Geometry check sheet. Reference: the model listing, model coordinates, mm. A direction names the side the tool comes from. Round coordinates to 2 decimals unless told otherwise and drop trailing zeros. Order: outer loops, then holes, each group sorted by start corner. A loop starts at its lowest first (then second) coordinate and runs counter-clockwise, first axis right, second up. Notation, with made-up numbers: (66, 52) -> (104, 52) arc R24 cw to (104, 79) -> close; hole circle Ø8 at (50, 77). An arc over 180 degrees is marked (long way). Answer as a JSON object with one key per item and string values. Group by question number.
from build123d import *

# Parameters (mm, degrees)
SKETCH_1_W          = 32
SKETCH_1_H          = 28
EXTRUDE_1_DEPTH     = 1.2
SKETCH_2_W          = 32
SKETCH_2_H          = 17.6
EXTRUDE_2_DEPTH     = 1.8
SKETCH_3_R          = 1.1
CUT_EXTRUDE_1_DEPTH = 43.558665393
SKETCH_4_R          = 0.4
EXTRUDE_3_DEPTH     = 10
SKETCH_5_W          = 20.3
SKETCH_5_H          = 2.5
EXTRUDE_4_DEPTH     = 2.5


with BuildPart() as part:
    # 草图1 → 凸台-拉伸1 (new body)
    with BuildSketch(Plane(origin=(0, 0, 0), x_dir=(1, 0, 0), z_dir=(0, 1, 0))):
        with Locations((16, 14)):
            Rectangle(SKETCH_1_W, SKETCH_1_H)
    extrude(amount=EXTRUDE_1_DEPTH)

    # 草图2 → 凸台-拉伸2 (add)
    with BuildSketch(Plane(origin=(0, 1.2, 0), x_dir=(1, 0, 0), z_dir=(0, 1, 0))):
        with Locations((16, 14)):
            Rectangle(SKETCH_2_W, SKETCH_2_H)
    extrude(amount=EXTRUDE_2_DEPTH)

    # 草图3 → 切除-拉伸1 (cut, through all)
    with BuildSketch(Plane(origin=(0, 1.2, 0), x_dir=(1, 0, 0), z_dir=(0, 1, 0))):
        with Locations(Location((2.75, 25.5, 0), (0, 0, 270))):
            Circle(SKETCH_3_R)
        with Locations(Location((2.75, 2.5, 0), (0, 0, 90))):
            Circle(SKETCH_3_R)
        with Locations(Location((29.25, 2.5, 0), (0, 0, 270))):
            Circle(SKETCH_3_R)
        with Locations(Location((29.25, 25.5, 0), (0, 0, 90))):
            Circle(SKETCH_3_R)
    extrude(amount=-CUT_EXTRUDE_1_DEPTH, mode=Mode.SUBTRACT)

    # 草图4 → 凸台-拉伸3 (add)
    with BuildSketch(Plane.XZ):
        with Locations(Location((7.11, -1.27, 0), (0, 0, 270))):
            Circle(SKETCH_4_R)
        with Locations(Location((9.65, -1.27, 0), (0, 0, 270))):
            Circle(SKETCH_4_R)
        with Locations(Location((12.19, -1.27, 0), (0, 0, 270))):
            Circle(SKETCH_4_R)
        with Locations(Location((14.73, -1.27, 0), (0, 0, 270))):
            Circle(SKETCH_4_R)
        with Locations(Location((17.27, -1.27, 0), (0, 0, 270))):
            Circle(SKETCH_4_R)
        with Locations(Location((19.81, -1.27, 0), (0, 0, 270))):
            Circle(SKETCH_4_R)
        with Locations(Location((22.35, -1.27, 0), (0, 0, 270))):
            Circle(SKETCH_4_R)
        with Locations(Location((24.89, -1.27, 0), (0, 0, 270))):
            Circle(SKETCH_4_R)
    extrude(amount=EXTRUDE_3_DEPTH)

    # 草图5 → 凸台-拉伸4 (add)
    with BuildSketch(Plane.XZ):
        with Locations((16, -1.25)):
            Rectangle(SKETCH_5_W, SKETCH_5_H)
    extrude(amount=EXTRUDE_4_DEPTH)


solid = part.part
Item 1: Mould release check, pull along X, two halves, no side actions. Record for faces 1 (the flat face through (26.15, -1, -1)), 2 (the cylindrical face through (10.047, -6.198, -1.218)), 3 (the flat face through (5.85, -1, -1)), 4 (the flat face through (16, 0, 0)): pulls with the +X half, pulls with the -X half, needs draft (parallel to the pull), parting line crosses it, or undercut.
Item 2: Sectioned sample at D-D, the plane x = 12.19. Enter the section's corners in (y, z).
Item 3: Set-up check for faces 5 (the flat face through (16, 2, -22.8)), 6 (the cylindrical face through (2.8, 0.6, -26.6)), 7 (the flat face through (16, -1, -2.5)), 8 (the cylindrical face through (15.127, -6.198, -1.218)), 9 (the flat face through (16, 1.2, -3)): record each of +Z, -Z, +X, -X, +Y, -Y from which the full face is reachable in a straight line by a thin tool's end or side.
Item 4: Sectioned sample at B-B, the plane y = -6.25. Enter the section's corners in (x, z).
Item 5: Depth check by flat-ended pin: pin 1 Ø1.2 at (y, z) = (-1, -2) entering from +X; pin 2 Ø3.5 at (x, z) = (29.25, -2.5) entering from +Y; pin 3 Ø10 at (x, z) = (8, -8) entering from -Y. Enter the tip coordinate at first touch or a pass-through.
Item 6: Thickness scan on L1, parallel to X at y = 0.75, z = -25.5; L2, parallel to Y at x = 13, z = -11.5; L3, parallel to Z at x = 10.5, y = 1.5. Record the ranges inside material, lowest first.
Item 7: Sectioned sample at A-A, the plane x = 29.25. Enter the section's corners in (y, z).
Item 8: Sectioned sample at C-C, the plane z = -25.5. Enter the section's corners in (x, y).
Result:
{
 "1": {"face 1": "pulls with the +X half", "face 2": "undercut", "face 3": "pulls with the -X half", "face 4": "needs draft"},
 "2": {"outline": "(-10, -1.67) -> (-2.5, -1.67) -> (-2.5, -2.5) -> (0, -2.5) -> (0, -28) -> (1.2, -28) -> (1.2, -22.8) -> (3, -22.8) -> (3, -5.2) -> (1.2, -5.2) -> (1.2, 0) -> (-2.5, 0) -> (-2.5, -0.87) -> (-10, -0.87) -> close"},
 "3": {"face 5": "-Z, +X, -X, +Y", "face 6": "+Y, -Y", "face 7": "-Z, +X, -X, -Y", "face 8": "-Y", "face 9": "+Z, +X, -X, +Y"},
 "4": {"outline": "circle Ø0.8 at (7.11, -1.27); circle Ø0.8 at (9.65, -1.27); circle Ø0.8 at (12.19, -1.27); circle Ø0.8 at (14.73, -1.27); circle Ø0.8 at (17.27, -1.27); circle Ø0.8 at (19.81, -1.27); circle Ø0.8 at (22.35, -1.27); circle Ø0.8 at (24.89, -1.27)"},
 "5": {"pin 1": "stops at x = 26.15", "pin 2": "stops at y = 1.2", "pin 3": "stops at y = 0"},
 "6": {"L1": "x = 0 to 1.65, 3.85 to 28.15, 30.35 to 32", "L2": "y = 0 to 3", "L3": "z = -22.8 to -5.2"},
 "7": {"outline": "(0, -28) -> (1.2, -28) -> (1.2, -26.6) -> (0, -26.6) -> close; (0, -24.4) -> (1.2, -24.4) -> (1.2, -22.8) -> (3, -22.8) -> (3, -5.2) -> (1.2, -5.2) -> (1.2, -3.6) -> (0, -3.6) -> close; (0, -1.4) -> (1.2, -1.4) -> (1.2, 0) -> (0, 0) -> close"},
 "8": {"outline": "(0, 0) -> (1.65, 0) -> (1.65, 1.2) -> (0, 1.2) -> close; (3.85, 0) -> (28.15, 0) -> (28.15, 1.2) -> (3.85, 1.2) -> close; (30.35, 0) -> (32, 0) -> (32, 1.2) -> (30.35, 1.2) -> close"}
}
